from build123d import *

# Parameters (mm, degrees)
BOSS_EXTRUDE1_DEPTH = 20
SKETCH2_R           = 1.400281721
BOSS_EXTRUDE3_DEPTH = 15


with BuildPart() as part:
    # Sketch1 → Boss-Extrude1 (new body)
    with BuildSketch(Plane.XY):
        with BuildLine():
            Line((3.102637299, 3.697579148), (4.279619218, 4.373206779))
            ThreePointArc((4.279619218, 4.373206779), (5.288327072, 3.077933555), (5.916340543, 1.561087044))
            Line((5.916340543, 1.561087044), (4.753516124, 0.838173146))
            Line((4.753516124, 0.838173146), (6.089421653, 0.599184544))
            ThreePointArc((6.089421653, 0.599184544), (6.029551119, -1.041437222), (5.535627206, -2.607088341))
            Line((5.535627206, -2.607088341), (4.180171925, -2.413423386))
            Line((4.180171925, -2.413423386), (5.04991602, -3.455202798))
            ThreePointArc((5.04991602, -3.455202798), (3.949481187, -4.673507948), (2.564732378, -5.555378116))
            Line((2.564732378, -5.555378116), (1.650878825, -4.535752294))
            Line((1.650878825, -4.535752294), (1.647498557, -5.892862351))
            ThreePointArc((1.647498557, -5.892862351), (0.021405114, -6.118792365), (-1.606229234, -5.90424473))
            Line((-1.606229234, -5.90424473), (-1.650878825, -4.535752294))
            Line((-1.650878825, -4.535752294), (-2.52580179, -5.573186118))
            ThreePointArc((-2.52580179, -5.573186118), (-3.91668665, -4.701025832), (-5.025618336, -3.490449616))
            Line((-5.025618336, -3.490449616), (-4.180171925, -2.413423386))
            Line((-4.180171925, -2.413423386), (-5.517251408, -2.645754161))
            ThreePointArc((-5.517251408, -2.645754161), (-6.022117201, -1.083597066), (-6.093464765, 0.556565665))
            Line((-6.093464765, 0.556565665), (-4.753516124, 0.838173146))
            Line((-4.753516124, 0.838173146), (-5.927117776, 1.519655572))
            ThreePointArc((-5.927117776, 1.519655572), (-5.309732185, 3.04085881), (-4.310111309, 4.343157686))
            Line((-4.310111309, 4.343157686), (-3.102637299, 3.697579148))
            Line((-3.102637299, 3.697579148), (-3.563619863, 4.974001574))
            ThreePointArc((-3.563619863, 4.974001574), (-2.112864469, 5.742463053), (-0.51000887, 6.097537957))
            Line((-0.51000887, 6.097537957), (0, 4.826846773))
            Line((0, 4.826846773), (0.467335389, 6.100956959))
            ThreePointArc((0.467335389, 6.100956959), (2.072636014, 5.757105014), (3.528732387, 4.998812451))
            Line((3.528732387, 4.998812451), (3.102637299, 3.697579148))
        make_face()
    extrude(amount=BOSS_EXTRUDE1_DEPTH)

    # Sketch2 → Boss-Extrude3 (add)
    with BuildSketch(Plane.XY.offset(20)):
        Circle(SKETCH2_R)
    extrude(amount=BOSS_EXTRUDE3_DEPTH)


solid = part.part
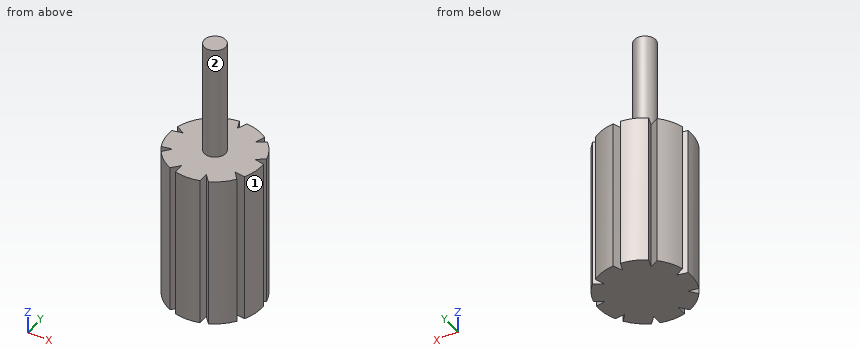
Can you work these out from the model? Positions are in its coordinate system, mm. Face numbers are marked on the shaded views. A direction names the side the tool comes from. Coordinates: 2 decimals unless noted, no trailing zeros. Write each loop counter-clockwise with the first axis right and the second up, starting at its lowest first coordinate (ties: lowest second). Pieces come first, ordered by that corner, then holes. Notation, with made-up numbers: (87, -31) - (112, -31) arc R11 cw to (112, -24) - close; hole circle Ø10 at (-35.75, 44). An arc over 180 degrees is marked (long way). Return JSON: item names as keys, results as strings. Group by question number.
Item 1: I'm going to push flat-ended pins straight in: pin 1 Ø4 at (x, z) = (-2, 14.5) entering from +Y; pin 2 Ø1.5 at (x, y) = (-3.5, 2) entering from +Z; pin 3 Ø3 at (y, z) = (3, 19.5) entering from +X. Where does each tip first touch, or does it pass through?
Item 2: If we section it at B-B (y = 0): Write out the boundary of the cut face in (x, z).
Item 3: Please list where these lines run through material, in increasing order: probe 1 along Z at (x, y) = (2.75, 0); probe 2 along X at (y, z) = (4, 12); probe 3 along X at (y, z) = (-4.25, 16).
Item 4: If we section it at D-D (y = 3): Write out the boundary of the cut face in (x, z), then the cut area to 3 significant figures.
Item 5: If we section it at A-A (z = 5.5): Write out the boundary of the cut face in (x, y), then the cut area to 3 significant figures.
Item 6: Which directions (+Z, -Z, +X, -X, +Y, -Y) give clear straight access to the entire face, cutting with the end or side of a thin tool? Please do the marked faces 1 and 2.
Item 7: If we section it at C-C (z = 29): Write out the boundary of the cut face in (x, y), then the cut area to 3 significant figures.
Return value:
{
 "1": {"pin 1": "stops at y = 6.1", "pin 2": "stops at z = 20", "pin 3": "stops at x = 5.92"},
 "2": {"outline": "(-6.12, 0) - (6.12, 0) - (6.12, 20) - (1.4, 20) - (1.4, 35) - (-1.4, 35) - (-1.4, 20) - (-6.12, 20) - close"},
 "3": {"probe 1": "z = 0 to 20", "probe 2": "x = -4.63 to -3.67, -3.21 to 3.2, 3.63 to 4.63", "probe 3": "x = -4.4 to 4.4"},
 "4": {"outline": "(-5.33, 0) - (5.33, 0) - (5.33, 20) - (-5.33, 20) - close", "area": "213 mm^2"},
 "5": {"outline": "(-6.09, 0.56) arc R6.12 ccw to (-5.52, -2.65) - (-4.18, -2.41) - (-5.03, -3.49) arc R6.12 ccw to (-2.53, -5.57) - (-1.65, -4.54) - (-1.61, -5.9) arc R6.12 ccw to (1.65, -5.89) - (1.65, -4.54) - (2.56, -5.56) arc R6.12 ccw to (5.05, -3.46) - (4.18, -2.41) - (5.54, -2.61) arc R6.12 ccw to (6.09, 0.6) - (4.75, 0.84) - (5.92, 1.56) arc R6.12 ccw to (4.28, 4.37) - (3.1, 3.7) - (3.53, 5) arc R6.12 ccw to (0.47, 6.1) - (0, 4.83) - (-0.51, 6.1) arc R6.12 ccw to (-3.56, 4.97) - (-3.1, 3.7) - (-4.31, 4.34) arc R6.12 ccw to (-5.93, 1.52) - (-4.75, 0.84) - close", "area": "112 mm^2"},
 "6": {"face 1": "+Z, -Z, +X", "face 2": "+Z"},
 "7": {"outline": "circle Ø2.8 at (0, 0)", "area": "6.16 mm^2"}
}
